For this review, take the finished solid that the model builds, in its own axes (mm). Face numbers are marked on the shaded views. Coordinates: 2 decimals unless noted, no trailing zeros. Loops run counter-clockwise (first coordinate to the right, second up) from the corner with the lowest first, then second, coordinate; pieces in that order, holes last. Notation, with made-up numbers: M -11,-33.75 L 20,-33.75 A29 cw 20,-1.75 Z; hole C 75.5,68 d7. An arc over 180 degrees is marked long. Answer as a JSON object with one key per item and string values. Group by question number.
Item 1: Add section B-B (x = 0). State the section outline as (y, z) points.
Item 2: Add section A-A (y = 104). State the section outline as (x, z) points, then the cut area to 3 significant figures.
Item 3: Mouldability with a two-part tool opening along Y and no side actions: class the marked faces 1, 2, 3 and 4 as +Y half, -Y half, draft (parallel to the pull), parting line (faces both ways), or undercut.
Item 4: Add section C-C (y = 147). State the section outline as (x, z) points.
Item 5: Insertion check: pin 1 (3 mm diameter, centred on x = 0.5, z = -12.5, fed in from +Y); pin 2 (1 mm diameter, centred on x = -12.5, z = -15, fed in from -Y); pin 3 (3.5 mm diameter, centred on x = -10, y = 16, fed in from -Z); pin 4 (3 mm diameter, centred on y = 76, z = -24, fed in from -X). Each pin has a flat end and moves straight along its axis. Give the tip position at first contact, or say it passes through.
Item 6: Wall thickness on L1, parallel to Y at x = 10, z = -17.5; L2, parallel to X at y = 16, z = -18.5; L3, parallel to Y at x = 11, z = -27.75: over which ranges is each line inside the solid? List them lowest first. Write a range as from..to.
Item 7: Add section D-D (y = 40). State the section outline as (x, z) points, then the cut area to 3 significant figures.
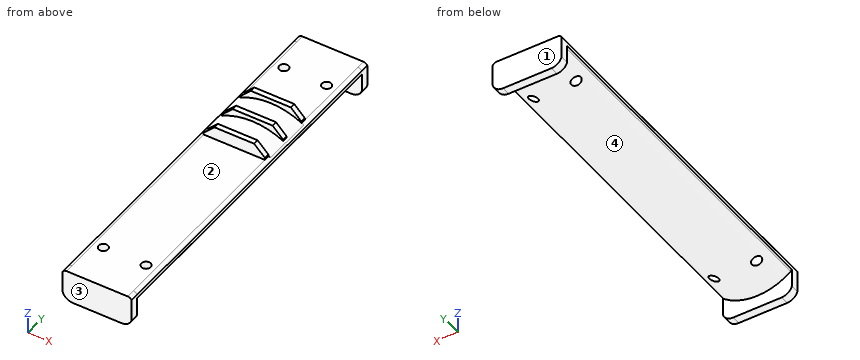
from build123d import *

# Parameters (mm, degrees)
BOSS_EXTRUDE1_DEPTH        = 163
FILLET1_R                  = 2
BOSS_EXTRUDE3_START        = 4
BOSS_EXTRUDE3_DEPTH        = 4
BOSS_EXTRUDE4_START        = -163
BOSS_EXTRUDE4_DEPTH        = 4
FILLET2_R                  = 5
BOSS_EXTRUDE5_START        = -126
BOSS_EXTRUDE5_DEPTH        = 24
SKETCH4_W                  = 28.635642126
SKETCH4_H                  = 6
BOSS_EXTRUDE6_DEPTH        = 2.5
BOSS_EXTRUDE7_START        = -24
SKETCH4_2_W                = 28.635642126
SKETCH4_2_H                = 6
BOSS_EXTRUDE7_DEPTH        = 2.5
BOSS_EXTRUDE8_DEPTH        = 1.25
BOSS_EXTRUDE8_DEPTH_BACK   = 1.25
BOSS_EXTRUDE8_START        = -12
SKETCH4_3_W                = 28.635642126
SKETCH4_3_H                = 6
CHAMFER1_SIZE              = 5
F_4_4_4_4_DIAMETER_HOLE1_D = 4.4
SKETCH7_W                  = 27.737228758
SKETCH7_H                  = 178.87682219
CUT_EXTRUDE1_DEPTH         = 0.2
CUT_EXTRUDE2_START         = -32.635642
SKETCH7_2_W                = 27.737228758
SKETCH7_2_H                = 178.87682219
CUT_EXTRUDE2_DEPTH         = 0.2


with BuildPart() as part:
    # Sketch1 → Boss-Extrude1 (new body)
    with BuildSketch(Plane(origin=(0, 0, 0), x_dir=(1, 0, 0), z_dir=(0, 1, 0))):
        with BuildLine():
            Line((-19.209372712, 16), (19.209372712, 16))
            ThreePointArc((19.209372712, 16), (0, 25), (-19.209372712, 16))
        make_face()
    extrude(amount=BOSS_EXTRUDE1_DEPTH)

    # Fillet1
    fillet1_edges = [part.edges().sort_by_distance(p)[0] for p in [
        (19.209372712, 81.5, -16),
        (-19.209372712, 81.5, -16),
    ]]
    fillet(fillet1_edges, radius=FILLET1_R)

    # Sketch2 → Boss-Extrude3 (add)
    with BuildSketch(Plane(origin=(0, 163, 0), x_dir=(1, 0, 0), z_dir=(0, 1, 0)).offset(BOSS_EXTRUDE3_START)):
        with BuildLine():
            Line((-16.317821063, 31), (-16.317821063, 18))
            ThreePointArc((-16.317821063, 18), (-15.732034626, 16.585786438), (-14.317821063, 16))
            Line((-14.317821063, 16), (14.317821063, 16))
            ThreePointArc((14.317821063, 16), (15.732034626, 16.585786438), (16.317821063, 18))
            Line((16.317821063, 18), (16.317821063, 31))
            Line((16.317821063, 31), (-16.317821063, 31))
        make_face()
    extrude(amount=-BOSS_EXTRUDE3_DEPTH)

    # Sketch2<2> → Boss-Extrude4 (add)
    with BuildSketch(Plane(origin=(0, 163, 0), x_dir=(1, 0, 0), z_dir=(0, 1, 0)).offset(BOSS_EXTRUDE4_START)):
        with BuildLine():
            Line((16.317821063, 31), (-16.317821063, 31))
            Line((-16.317821063, 31), (-16.317821063, 18))
            ThreePointArc((-16.317821063, 18), (-16.119217166, 18.868891294), (-15.562848982, 19.565217391))
            ThreePointArc((-15.562848982, 19.565217391), (0, 25), (15.562848982, 19.565217391))
            ThreePointArc((15.562848982, 19.565217391), (16.119217166, 18.868891294), (16.317821063, 18))
            Line((16.317821063, 18), (16.317821063, 31))
        make_face()
        with BuildLine():
            ThreePointArc((-15.562848982, 19.565217391), (-16.119217166, 18.868891294), (-16.317821063, 18))
            ThreePointArc((-16.317821063, 18), (-15.732034626, 16.585786438), (-14.317821063, 16))
            Line((-14.317821063, 16), (14.317821063, 16))
            ThreePointArc((14.317821063, 16), (15.732034626, 16.585786438), (16.317821063, 18))
            ThreePointArc((16.317821063, 18), (16.119217166, 18.868891294), (15.562848982, 19.565217391))
            ThreePointArc((15.562848982, 19.565217391), (0, 25), (-15.562848982, 19.565217391))
        make_face()
    extrude(amount=-BOSS_EXTRUDE4_DEPTH)

    # Fillet2
    fillet2_edges = [part.edges().sort_by_distance(p)[0] for p in [
        (16.317821063, 165, -31),
        (-16.317821063, 165, -31),
        (16.317821063, -2, -31),
        (-16.317821063, -2, -31),
    ]]
    fillet(fillet2_edges, radius=FILLET2_R)

    # Sketch3 → Boss-Extrude5 (add)
    with BuildSketch(Plane.XZ.offset(4).offset(BOSS_EXTRUDE5_START)):
        with BuildLine():
            ThreePointArc((15.340522568, -16.281255798), (0, -12.062418831), (-15.340522568, -16.281255798))
            ThreePointArc((-15.340522568, -16.281255798), (-14.848156615, -16.071595426), (-14.317821063, -16))
            Line((-14.317821063, -16), (14.317821063, -16))
            ThreePointArc((14.317821063, -16), (14.848156615, -16.071595426), (15.340522568, -16.281255798))
        make_face()
    extrude(amount=BOSS_EXTRUDE5_DEPTH)

    # Sketch4 → Boss-Extrude6 (add)
    with BuildSketch(Plane(origin=(0, 122, 0), x_dir=(1, 0, 0), z_dir=(0, 1, 0))):
        with Locations((0, 13)):
            Rectangle(SKETCH4_W, SKETCH4_H)
    extrude(amount=BOSS_EXTRUDE6_DEPTH)

    # Sketch4<2> → Boss-Extrude7 (add)
    with BuildSketch(Plane(origin=(0, 122, 0), x_dir=(1, 0, 0), z_dir=(0, 1, 0)).offset(BOSS_EXTRUDE7_START)):
        with Locations((0, 13)):
            Rectangle(SKETCH4_2_W, SKETCH4_2_H)
    extrude(amount=-BOSS_EXTRUDE7_DEPTH)

    # Sketch4<3> → Boss-Extrude8 (add, two sides: drawn at the far end of the back side and taken through both)
    with BuildSketch(Plane(origin=(0, 122, 0), x_dir=(1, 0, 0), z_dir=(0, 1, 0)).offset(BOSS_EXTRUDE8_START - BOSS_EXTRUDE8_DEPTH_BACK)):
        with Locations((0, 13)):
            Rectangle(SKETCH4_3_W, SKETCH4_3_H)
    extrude(amount=BOSS_EXTRUDE8_DEPTH + BOSS_EXTRUDE8_DEPTH_BACK)

    # Chamfer1
    chamfer1_edges = [part.edges().sort_by_distance(p)[0] for p in [
        (-14.317821063, 123.25, -10),
        (14.317821063, 123.25, -10),
        (14.317821063, 96.75, -10),
        (-14.317821063, 96.75, -10),
        (-14.317821063, 110, -10),
        (14.317821063, 110, -10),
    ]]
    chamfer(chamfer1_edges, length=CHAMFER1_SIZE)

    # Ø4.4 (4.4) Diameter Hole1 (through all)
    with Locations(Plane.XY.offset(-16)):
        with Locations((-10, 147), (10, 147), (10, 16), (-10, 16)):
            Hole(F_4_4_4_4_DIAMETER_HOLE1_D / 2)

    # Sketch7 → Cut-Extrude1 (cut)
    with BuildSketch(Plane.ZY.offset(16.317821063)):
        with Locations((-24.632131786, 79.951369179)):
            Rectangle(SKETCH7_W, SKETCH7_H)
    extrude(amount=-CUT_EXTRUDE1_DEPTH, mode=Mode.SUBTRACT)

    # Sketch7<2> → Cut-Extrude2 (cut)
    with BuildSketch(Plane.ZY.offset(16.317821063).offset(CUT_EXTRUDE2_START)):
        with Locations((-24.632131786, 79.951369179)):
            Rectangle(SKETCH7_2_W, SKETCH7_2_H)
    extrude(amount=CUT_EXTRUDE2_DEPTH, mode=Mode.SUBTRACT)


solid = part.part
From the geometry:
{
 "1": {"outline": "M -4,-31 L 0,-31 L 0,-25 L 163,-25 L 163,-31 L 167,-31 L 167,-16 L 124.5,-16 L 124.5,-10 L 122,-10 L 122,-12.06 L 111.25,-12.06 L 111.25,-10 L 108.75,-10 L 108.75,-12.06 L 98,-12.06 L 98,-10 L 95.5,-10 L 95.5,-16 L -4,-16 Z"},
 "2": {"outline": "M -16.12,-18.87 A2 ccw -15.56,-19.57 A25 ccw 15.56,-19.57 A2 ccw 16.12,-18.87 L 16.12,-17.13 A2 ccw 15.34,-16.28 A30 ccw -15.34,-16.28 A2 ccw -16.12,-17.13 Z", "area": "308 mm²"},
 "3": {"face 1": "+Y half", "face 2": "draft", "face 3": "-Y half", "face 4": "undercut"},
 "4": {"outline": "M -16.12,-18.87 A2 ccw -15.56,-19.57 A25 ccw -12.2,-21.82 L -12.2,-16 L -14.32,-16 A2 ccw -16.12,-17.13 Z; M -7.8,-23.75 A25 ccw 7.8,-23.75 L 7.8,-16 L -7.8,-16 Z; M 12.2,-21.82 A25 ccw 15.56,-19.57 A2 ccw 16.12,-18.87 L 16.12,-17.13 A2 ccw 14.32,-16 L 12.2,-16 Z"},
 "5": {"pin 1": "stops at y = 124.5", "pin 2": "stops at y = 95.5", "pin 3": "passes through", "pin 4": "stops at x = -10.9"},
 "6": {"L1": "y = -4..13.8, 18.2..144.8, 149.2..167", "L2": "x = -16.12..-12.2, -7.8..7.8, 12.2..16.12", "L3": "y = -4..0, 163..167"},
 "7": {"outline": "M -16.12,-18.87 A2 ccw -15.56,-19.57 A25 ccw 15.56,-19.57 A2 ccw 16.12,-18.87 L 16.12,-17.13 A2 ccw 14.32,-16 L -14.32,-16 A2 ccw -16.12,-17.13 Z", "area": "229 mm²"}
}
